Verification items for the finished model (mm, model axes). A direction names the side the tool comes from. Give positions to 0.01 mm unless a question says otherwise; leave off trailing zeros. Order: outer loops, then holes, each group sorted by start corner. A loop starts at its lowest first (then second) coordinate and runs counter-clockwise, first axis right, second up.
(1) Mould release check, pull along Z, two halves, no side actions. Record for faces 5 (the face through (15.836, 3.549, -12.825)), 6 (the face through (93.3, 19, -41)), 7 (the face through (1, 9, -2)): pulls with the +Z half, pulls with the -Z half, needs draft (parallel to the pull), parting line crosses it, or undercut.
(2) Sectioned sample at C-C on x = 69.24. Record the cut outline in (y, z).
(3) Scan lines: L1, parallel to X at y = 15, z = -5; L2, parallel to Z at x = 90, y = 15.5; L3, parallel to Z at x = 14.5, y = 14.75. Record each from-to range of solid material in increasing order.
(4) Gauge pin test, flat ends, axial feed: pin 1 (1.8 mm diameter, centred on x = 18.5, z = -14, fed in from +Y); pin 2 (5 mm diameter, centred on x = 13.5, z = -19.5, fed in from +Y); pin 3 (0.9 mm diameter, centred on x = 1, y = 15.5, fed in from +Z). Record the tip position at first contact, or that the pin passes through.
(5) Sectioned sample at A-A on y = 11.25. Count the separate pieces of the cut face and the enclosed holes in it, plus the area to 3 significant figures.
(6) Sectioned sample at B-B on z = -45.52. Record the cut outline in (x, y).
(7) Access from +Z, -Z, +X, -X, +Y, -Y to the whole of each face (thin tool, end or side, straight path). Record for faces 1 (the face through (1.7, 19, -66)), 2 (the face through (47, 19, -1.7)), 3 (the face through (2, 14, -41.75)), 4 (the face through (6, 11, -74)).
```python
from build123d import *

# Parameters (mm, degrees)
SKETCH1_W           = 95
SKETCH1_H           = 83
BOSS_EXTRUDE1_DEPTH = 3
SKETCH2_W           = 95
SKETCH2_H           = 83
SKETCH2_W_2         = 89
SKETCH2_H_2         = 77
BOSS_EXTRUDE2_DEPTH = 17
SKETCH4_R           = 3
BOSS_EXTRUDE3_DEPTH = 4
SKETCH5_R           = 1.5
CUT_EXTRUDE2_DEPTH  = 7
SKETCH6_W           = 6
SKETCH6_H           = 6
BOSS_EXTRUDE4_DEPTH = 17
SKETCH7_R           = 1.5
CUT_EXTRUDE3_DEPTH  = 20
FILLET4_R           = 5
CUT_EXTRUDE4_DEPTH  = 3
CUT_EXTRUDE1_REACH  = 127.511
SKETCH3_W           = 10
SKETCH3_H           = 11
SKETCH3_W_2         = 12.5


with BuildPart() as part:
    # Sketch1 → Boss-Extrude1 (new body)
    with BuildSketch(Plane(origin=(0, 0, 0), x_dir=(1, 0, 0), z_dir=(0, 1, 0))):
        with Locations((47.5, 41.5)):
            Rectangle(SKETCH1_W, SKETCH1_H)
    extrude(amount=BOSS_EXTRUDE1_DEPTH)

    # Sketch2 → Boss-Extrude2 (add)
    with BuildSketch(Plane(origin=(0, 3, 0), x_dir=(1, 0, 0), z_dir=(0, 1, 0))):
        with Locations((47.5, 41.5)):
            Rectangle(SKETCH2_W, SKETCH2_H)
        with Locations((47.5, 41.5)):
            Rectangle(SKETCH2_W_2, SKETCH2_H_2, mode=Mode.SUBTRACT)
    extrude(amount=BOSS_EXTRUDE2_DEPTH)

    # Sketch4 → Boss-Extrude3 (add)
    with BuildSketch(Plane(origin=(0, 3, 0), x_dir=(1, 0, 0), z_dir=(0, 1, 0))):
        with Locations(Location((17.3, 12.5, 0), (0, 0, 90))):
            Circle(SKETCH4_R)
        with Locations(Location((18.57, 60.76, 0), (0, 0, 90))):
            Circle(SKETCH4_R)
        with Locations(Location((69.24, 45.52, 0), (0, 0, 90))):
            Circle(SKETCH4_R)
        with Locations(Location((69.24, 17.58, 0), (0, 0, 90))):
            Circle(SKETCH4_R)
    extrude(amount=BOSS_EXTRUDE3_DEPTH)

    # Sketch5 → Cut-Extrude2 (cut)
    with BuildSketch(Plane(origin=(0, 7, 0), x_dir=(1, 0, 0), z_dir=(0, 1, 0))):
        with Locations(Location((18.57, 60.76, 0), (0, 0, 270))):
            Circle(SKETCH5_R)
        with Locations(Location((69.24, 45.52, 0), (0, 0, 270))):
            Circle(SKETCH5_R)
        with Locations(Location((69.24, 17.58, 0), (0, 0, 270))):
            Circle(SKETCH5_R)
        with Locations(Location((17.3, 12.5, 0), (0, 0, 270))):
            Circle(SKETCH5_R)
    extrude(amount=-CUT_EXTRUDE2_DEPTH, mode=Mode.SUBTRACT)

    # Sketch6 → Boss-Extrude4 (add)
    with BuildSketch(Plane(origin=(0, 3, 0), x_dir=(1, 0, 0), z_dir=(0, 1, 0))):
        with Locations((6, 6)):
            Rectangle(SKETCH6_W, SKETCH6_H)
        with Locations((89, 6)):
            Rectangle(SKETCH6_W, SKETCH6_H)
        with Locations((89, 77)):
            Rectangle(SKETCH6_W, SKETCH6_H)
        with Locations((6, 77)):
            Rectangle(SKETCH6_W, SKETCH6_H)
    extrude(amount=BOSS_EXTRUDE4_DEPTH)

    # Sketch7 → Cut-Extrude3 (cut)
    with BuildSketch(Plane(origin=(0, 20, 0), x_dir=(1, 0, 0), z_dir=(0, 1, 0))):
        with Locations(Location((5, 5, 0), (0, 0, 270))):
            Circle(SKETCH7_R)
        with Locations(Location((90, 5, 0), (0, 0, 270))):
            Circle(SKETCH7_R)
        with Locations(Location((90, 78, 0), (0, 0, 270))):
            Circle(SKETCH7_R)
        with Locations(Location((5, 78, 0), (0, 0, 270))):
            Circle(SKETCH7_R)
    extrude(amount=-CUT_EXTRUDE3_DEPTH, mode=Mode.SUBTRACT)

    # Fillet4
    fillet4_edges = [part.edges().sort_by_distance(p)[0] for p in [
        (0, 10, -83),
        (95, 10, -83),
        (95, 10, 0),
        (0, 10, 0),
    ]]
    fillet(fillet4_edges, radius=FILLET4_R)

    # Sketch9 → Cut-Extrude4 (cut)
    with BuildSketch(Plane(origin=(0, 20, 0), x_dir=(1, 0, 0), z_dir=(0, 1, 0))):
        with BuildLine():
            Line((95, 5), (95, 78))
            ThreePointArc((95, 78), (93.535533906, 81.535533906), (90, 83))
            Line((90, 83), (5, 83))
            ThreePointArc((5, 83), (1.464466094, 81.535533906), (0, 78))
            Line((0, 78), (0, 5))
            ThreePointArc((0, 5), (1.464466094, 1.464466094), (5, 0))
            Line((5, 0), (90, 0))
            ThreePointArc((90, 0), (93.535533906, 1.464466094), (95, 5))
        make_face()
        with BuildLine():
            Line((93.3, 5), (93.3, 78))
            ThreePointArc((93.3, 78), (92.333452378, 80.333452378), (90, 81.3))
            Line((90, 81.3), (5, 81.3))
            ThreePointArc((5, 81.3), (2.666547622, 80.333452378), (1.7, 78))
            Line((1.7, 78), (1.7, 5))
            ThreePointArc((1.7, 5), (2.666547622, 2.666547622), (5, 1.7))
            Line((5, 1.7), (90, 1.7))
            ThreePointArc((90, 1.7), (92.333452378, 2.666547622), (93.3, 5))
        make_face(mode=Mode.SUBTRACT)
    extrude(amount=-CUT_EXTRUDE4_DEPTH, mode=Mode.SUBTRACT)

    # Cut-Extrude1: up to this face of the body (flat: up to its plane)
    cut_extrude1_end = Plane(part.part.faces().sort_by_distance((0, 8.5, -41.5))[0])
    # Sketch3 → Cut-Extrude1 (cut, up to the picked face)
    with BuildSketch(Plane(origin=(3, 0, 0), x_dir=(0, 0, -1), z_dir=(1, 0, 0)), mode=Mode.PRIVATE) as cut_extrude1_sk1:
        with Locations((17.75, 14.5)):
            Rectangle(SKETCH3_W, SKETCH3_H)
    cut_extrude1_tool1 = split(extrude(cut_extrude1_sk1.sketch, amount=-CUT_EXTRUDE1_REACH, mode=Mode.PRIVATE), bisect_by=cut_extrude1_end, keep=Keep.BOTH, mode=Mode.PRIVATE)
    # Sketch3 → Cut-Extrude1 (cut, up to the picked face)
    with BuildSketch(Plane(origin=(3, 0, 0), x_dir=(0, 0, -1), z_dir=(1, 0, 0)), mode=Mode.PRIVATE) as cut_extrude1_sk2:
        with Locations((48, 14.5)):
            Rectangle(SKETCH3_W_2, SKETCH3_H)
    cut_extrude1_tool2 = split(extrude(cut_extrude1_sk2.sketch, amount=-CUT_EXTRUDE1_REACH, mode=Mode.PRIVATE), bisect_by=cut_extrude1_end, keep=Keep.BOTH, mode=Mode.PRIVATE)
    add(cut_extrude1_tool1.solids().sort_by(Axis((3, 14.5, -17.75), (-1, 0, 0)))[0], mode=Mode.SUBTRACT)
    add(cut_extrude1_tool2.solids().sort_by(Axis((3, 14.5, -48), (-1, 0, 0)))[0], mode=Mode.SUBTRACT)


solid = part.part
```
Ans:
1. face 5: undercut
1. face 6: needs draft
1. face 7: pulls with the +Z half
2. outline: (0, -83) - (17, -83) - (17, -81.3) - (20, -81.3) - (20, -80) - (3, -80) - (3, -48.52) - (7, -48.52) - (7, -47.02) - (0, -47.02) - close; (0, -44.02) - (7, -44.02) - (7, -42.52) - (3, -42.52) - (3, -20.58) - (7, -20.58) - (7, -19.08) - (0, -19.08) - close; (0, -16.08) - (7, -16.08) - (7, -14.58) - (3, -14.58) - (3, -3) - (20, -3) - (20, -1.7) - (17, -1.7) - (17, 0) - (0, 0) - close
3. L1: x = 0 to 3.5, 6.5 to 9, 86 to 88.5, 91.5 to 95
3. L2: z = -83 to -79.5, -76.5 to -74, -9 to -6.5, -3.5 to 0
3. L3: z = -83 to -80, -3 to 0
4. pin 1: stops at y = 7
4. pin 2: stops at y = 3
4. pin 3: stops at z = -1.48
5. separate pieces: 2
5. enclosed holes: 4
5. area: 1,060 mm2
6. outline: (0, 0) - (67.74, 0) - (67.74, 7) - (66.24, 7) - (66.24, 3) - (3, 3) - (3, 9) - (0, 9) - close; (70.74, 0) - (95, 0) - (95, 17) - (93.3, 17) - (93.3, 20) - (92, 20) - (92, 3) - (72.24, 3) - (72.24, 7) - (70.74, 7) - close
7. face 1: +Z, -Z, -X, +Y
7. face 2: +Z, +X, -X, +Y
7. face 3: -X, +Y
7. face 4: +Y
